Input: dimensioned drawing with shaded views. Units: mm. Origin: part minimum x, y, z. Round coordinates to 2 decimals unless told otherwise and drop trailing zeros. Order: outer loops, then holes, each group sorted by start corner. A loop starts at its lowest first (then second) coordinate and runs counter-clockwise, first axis right, second up. Notation, with made-up numbers: (63, 30) - (72, 30) arc R27 cw to (72, 46) - close; hole circle Ø1 at (51, 20.25). An arc over 180 degrees is marked (long way). Put each result on its own line as item: value. Start each with the question number.
(1) Pin query (flat end, axial travel): P1, Ø2, axis at x = 16, z = 6, coming from the +Y side; P2, Ø7.5, axis at x = 14.5, z = 9, coming from the -Y side. Return the tip coordinate at first contact, or that it passes through.
(2) Section A-A (z = 10). Output: boundary loops of the cut face in (x, y) (3 decimals), and give its area (3 significant figures).
(3) Material intervals for L1, parallel to X at y = 239, z = 9.25 (3 decimals); L2, parallel to Y at x = 36.5, z = 11; L3, parallel to Z at x = 11.5, y = 110, sorted ascending. Write a range as [from, to].
(4) Section C-C (x = 34.5). Output: boundary loops of the cut face in (y, z), and give its area (3 significant figures).
(5) Section B-B (y = 181.5). Output: boundary loops of the cut face in (x, z) (3 decimals).
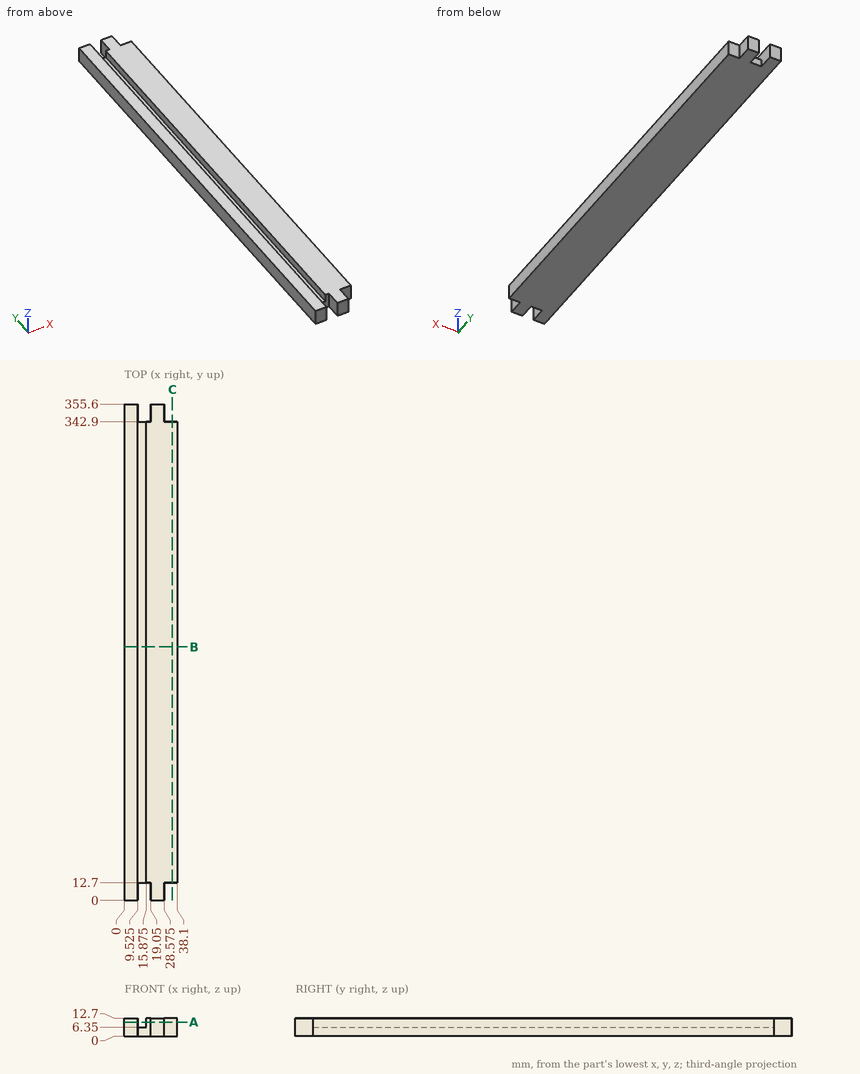
Checks:
1. P1: stops at y = 342.9
1. P2: stops at y = 12.7
2. outline: (0, 0) - (9.525, 0) - (9.525, 355.6) - (0, 355.6) - close; (15.875, 12.7) - (19.05, 12.7) - (19.05, 0) - (28.575, 0) - (28.575, 12.7) - (38.1, 12.7) - (38.1, 342.9) - (28.575, 342.9) - (28.575, 355.6) - (19.05, 355.6) - (19.05, 342.9) - (15.875, 342.9) - close
2. area: 11,000 mm²
3. L1: x = [0, 9.525], [15.875, 38.1]
3. L2: y = [12.7, 342.9]
3. L3: z = [0, 6.35]
4. outline: (12.7, 0) - (342.9, 0) - (342.9, 12.7) - (12.7, 12.7) - close
4. area: 4,190 mm²
5. outline: (0, 0) - (38.1, 0) - (38.1, 12.7) - (15.875, 12.7) - (15.875, 6.35) - (9.525, 6.35) - (9.525, 12.7) - (0, 12.7) - close
